Here's how the part is built. I have some questions about the finished solid (model axes, mm). A direction names the side the tool comes from. Round coordinates to 2 decimals unless told otherwise and drop trailing zeros. Order: outer loops, then holes, each group sorted by start corner. A loop starts at its lowest first (then second) coordinate and runs counter-clockwise, first axis right, second up. Notation, with made-up numbers: (86, 35) -> (98, 35) arc R25 cw to (98, 73) -> close; hole circle Ø9 at (6.25, 20). An arc over 180 degrees is marked (long way). Answer in a Markdown table with one row per item.
```python
from build123d import *

# Parameters (mm, degrees)
EXTRUDE_1_DEPTH        = 117.5
SKETCH_2_R             = 1.75
CUT_EXTRUDE_1_DEPTH    = 118.765657133
CHAMFER_1_SIZE         = 0.5
SKETCH_3_R             = 3.25
CUT_EXTRUDE_2_DEPTH    = 3.5
PATTERN_LINEAR_1_COUNT = 12
PATTERN_LINEAR_1_PITCH = 20


with BuildPart() as part:
    # 草图1 → 凸台-拉伸1 (new, symmetric)
    with BuildSketch(Plane.XY):
        Polygon((4.5, 0), (-4.5, 0), (-4.5, 3.292893219), (-4.042893219, 3.75), (-3.542893219, 3.75), (-3.542893219, 4.25), (-4.042893219, 4.25), (-4.5, 4.707106781), (-4.5, 6.5), (4.5, 6.5), (4.5, 4.707106781), (4.042893219, 4.25), (3.542893219, 4.25), (3.542893219, 3.75), (4.042893219, 3.75), (4.5, 3.292893219), align=None)
    extrude(amount=EXTRUDE_1_DEPTH, both=True)

    # 草图2 → 切除-拉伸1 (cut, through all)
    with BuildSketch(Plane(origin=(0, 6.5, 0), x_dir=(1, 0, 0), z_dir=(0, 1, 0))):
        with Locations(Location((0, 110, 0), (0, 0, 180))):
            Circle(SKETCH_2_R)
        with Locations(Location((0, 90, 0), (0, 0, 180))):
            Circle(SKETCH_2_R)
        with Locations(Location((0, 70, 0), (0, 0, 180))):
            Circle(SKETCH_2_R)
        with Locations(Location((0, 50, 0), (0, 0, 180))):
            Circle(SKETCH_2_R)
        with Locations(Location((0, 30, 0), (0, 0, 180))):
            Circle(SKETCH_2_R)
        with Locations(Location((0, 10, 0), (0, 0, 180))):
            Circle(SKETCH_2_R)
        with Locations(Location((0, -10, 0), (0, 0, 180))):
            Circle(SKETCH_2_R)
        with Locations(Location((0, -30, 0), (0, 0, 180))):
            Circle(SKETCH_2_R)
        with Locations(Location((0, -50, 0), (0, 0, 180))):
            Circle(SKETCH_2_R)
        with Locations(Location((0, -70, 0), (0, 0, 180))):
            Circle(SKETCH_2_R)
        with Locations(Location((0, -90, 0), (0, 0, 180))):
            Circle(SKETCH_2_R)
        with Locations(Location((0, -110, 0), (0, 0, 180))):
            Circle(SKETCH_2_R)
    extrude(amount=-CUT_EXTRUDE_1_DEPTH, mode=Mode.SUBTRACT)

    # 倒角1
    chamfer_1_edges = [part.edges().sort_by_distance(p)[0] for p in [
        (-4.5, 6.5, 0),
        (4.5, 6.5, 0),
        (4.5, 0, 0),
        (-4.5, 0, 0),
    ]]
    chamfer(chamfer_1_edges, length=CHAMFER_1_SIZE)

    # 草图3 → 切除-拉伸2 (cut)
    with BuildSketch(Plane(origin=(0, 6.5, 0), x_dir=(1, 0, 0), z_dir=(0, 1, 0))):
        with Locations(Location((0, 110, 0), (0, 0, 180))):
            Circle(SKETCH_3_R)
    cut_extrude_2 = extrude(amount=-CUT_EXTRUDE_2_DEPTH, mode=Mode.SUBTRACT)

    # 阵列(线性)1: 切除-拉伸2 ×12
    with Locations(*[(0, 0, i * PATTERN_LINEAR_1_PITCH) for i in range(1, PATTERN_LINEAR_1_COUNT)]):
        add(cut_extrude_2, mode=Mode.SUBTRACT)


solid = part.part
```
1. Suppose I cut it at A-A on y = 2. State how many separate pieces and enclosed holes the cut face has, then the cut area to 3 significant figures.
Numbers:
| item | result |
|---|---|
| separate pieces | 1 |
| enclosed holes | 12 |
| area | 2,000 mm2 |
2. Please list where these lines run through material, in increasing order: line 1 along X through (y, z) = (1.9, 90); line 2 along X through (y, z) = (5, 107.5); line 3 along X through (y, z) = (4.5, 59).
Numbers:
| item | result |
|---|---|
| line 1 | x = -4.5 to -1.75, 1.75 to 4.5 |
| line 2 | x = -4.5 to -2.08, 2.08 to 4.5 |
| line 3 | x = -4.29 to 4.29 |
3. For pin 1 Ø3 at (y, z) = (3.5, 22.5) entering from +X; pin 2 Ø4.5 at (x, z) = (0, -70) entering from +Y; pin 3 Ø0.6 at (y, z) = (4, -16) entering from -X, each with a flat end and sliding along its axis, tell me the tip position at first contact or that it passes through.
Numbers:
| item | result |
|---|---|
| pin 1 | stops at x = 4.5 |
| pin 2 | stops at y = 3 |
| pin 3 | stops at x = -4.09 |
4. For faces 5 (the face through (0.705, 4.774, -53.173)), 6 (the face through (0, 3, 117.5)), which set-ups out of +Z, -Z, +X, -X, +Y, -Y let a thin tool reach every point of the face, with its end or its side?
Numbers:
| item | result |
|---|---|
| face 5 | +Y |
| face 6 | +Z, +X, -X, +Y, -Y |
5. Suppose I cut it at B-B on z = 21. Write out the boundary of the cut face in (x, y).
Numbers:
| item | result |
|---|---|
| outline | (-4.5, 0.5) -> (-4, 0) -> (4, 0) -> (4.5, 0.5) -> (4.5, 3.29) -> (4.04, 3.75) -> (3.54, 3.75) -> (3.54, 4.25) -> (4.04, 4.25) -> (4.5, 4.71) -> (4.5, 6) -> (4, 6.5) -> (-4, 6.5) -> (-4.5, 6) -> (-4.5, 4.71) -> (-4.04, 4.25) -> (-3.54, 4.25) -> (-3.54, 3.75) -> (-4.04, 3.75) -> (-4.5, 3.29) -> close |
6. We'd pull the mould along Z, two halves only. Please class faces 1 (the face through (0, 3, -117.5)), 2 (the face through (-1.4, 3, 48.6)), 3 (the face through (0.705, 4.774, -113.173)), 4 (the face through (0, 0, 2)): released by +Z, released by -Z, zero draft, split by the parting line, or undercut.
Numbers:
| item | result |
|---|---|
| face 1 | released by -Z |
| face 2 | undercut |
| face 3 | undercut |
| face 4 | zero draft |
